Autodesk Inventor part; units mm, degrees
ref_plane "YZ Plane" through (0, 0, 0) normal (1, 0, 0) x (0, 1, 0)
ref_plane "XZ Plane" through (0, 0, 0) normal (0, 1, 0) x (-1, 0, 0)
ref_plane "XY Plane" through (0, 0, 0) normal (0, 0, 1) x (1, 0, 0)
sketch "Sketch1" plane through (0, 0, 0) normal (0, 1, 0) x (-1, 0, 0)
  circle A0 centre (0, 0) radius 14
  dimension "d0" = 28
extrude "Extrusion1" add sketch "Sketch1" along normal blind 50
sketch "Sketch2" plane through (0, 50, 0) normal (0, 1, 0) x (1, 0, 0)
  circle A0 centre (0, 0) radius 2.5
  dimension "d3" = 5
hole "Hole1" at (0, 50, 0) direction (0, -1, 0) diameter 10.106 depth 50 tip angle 118
sketch "Sketch3" plane through (0, 0, 0) normal (1, 0, 0) x (0, 1, 0)
  line L0 (50, -14) -> (50, 14)
  line L1 (50, 14.1595) -> (0, -14)
  line L2 (0, 14) -> (0, -14)
  line L3 (50, 14.1595) -> (50, -14)
  line L4 (0, 14.1595) -> (15, 14.1595)
  line L5 (15, 14.1595) -> (15, 0.0798)
  circle A0 centre (15, 0.0798) radius 2
  point P0 (0, 0)
  dimension "d11" = 15
  dimension "d12" = 4
hole "Hole2" at (0, 15, 0.0798) direction (-1, 0, 0) diameter 6.647 depth 22.2 tip angle 118
fillet "Fillet1" radius 5 1 edges at (14, 0, 0)
properties part number "FIXADOR_APOIO_ROLAMENTO"
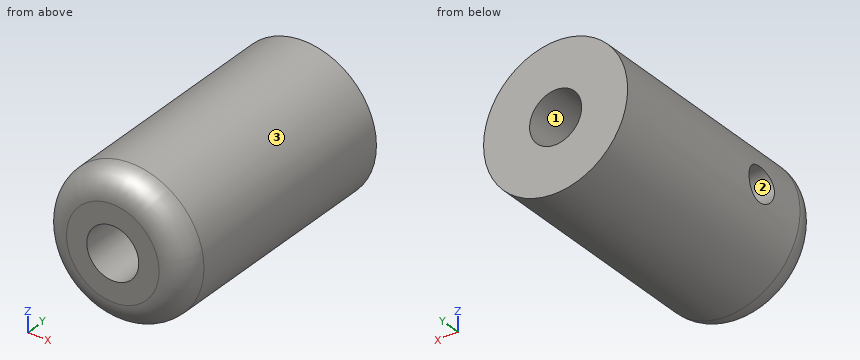
The listing builds one solid part. Answer for the finished solid, in the listing's coordinates (mm). Face numbers are marked on the shaded views. Round coordinates to 2 decimals unless told otherwise and drop trailing zeros. Order: outer loops, then holes, each group sorted by start corner. A loop starts at its lowest first (then second) coordinate and runs counter-clockwise, first axis right, second up. Notation, with made-up numbers: (31, 39.25) - (87, 39.25) arc R18 cw to (87, 56.25) - close; hole circle Ø10 at (23.25, 43). An arc over 180 degrees is marked (long way). Write item = value, one per line. Start each with the question number.
1) Straight lines are drawn through the part: L1, parallel to Z at x = 0, y = 18.5; L2, parallel to X at y = 3.5, z = -1.5; L3, parallel to Z at x = -7.5, y = 15. For each, find the intervals that lie inside material, in ascending order.
2) For a pull along X with two mould halves and no side action, classify the marked faces 1, 2 and 3 as released by +X, released by -X, zero draft, split by the parting line, or undercut.
3) Section C-C, the plane y = 24 is taken. Write down the section's boundary in (x, z).
4) Section B-B, the plane z = 0 is taken. Write down the section's boundary in (x, y).
5) Given pin 1 (6 mm diameter, centred on y = 30, z = -2.5, fed in from -X); pin 2 (4 mm diameter, centred on x = 9.5, z = 6.5, fed in from -Y); pin 3 (1 mm diameter, centred on x = -10, z = -6, fed in from -Y); pin 4 (5 mm diameter, centred on x = -3, y = 35.5, fed in from -Z), each flat-ended and moving along its own axis, determine where each tip first touches the part or whether it passes through.
6) Section D-D, the plane y = 15 is taken. Write down the section's boundary in (x, z).
7) Section A-A, the plane x = 0 is taken. Write down the section's boundary in (y, z), plus the area to 3 significant figures.
Results list:
q1.L1 = -14 to -5.05, 5.05 to 14
q1.L2 = -13.69 to -4.83, 4.83 to 13.69
q1.L3 = -11.82 to -3.24, 3.4 to 11.82
q2.face_1 = undercut
q2.face_2 = zero draft
q2.face_3 = split by the parting line
q3.outline = circle Ø28 at (0, 0); hole circle Ø10.11 at (0, 0)
q4.outline = (-14, 5) arc R5 ccw to (-9, 0) - (-5.05, 0) - (-5.05, 11.68) - (-14, 11.68) - close; (-14, 18.32) - (-5.05, 18.32) - (-5.05, 50) - (-14, 50) - close; (5.05, 0) - (9, 0) arc R5 ccw to (14, 5) - (14, 50) - (5.05, 50) - close
q5.pin_1 = -14
q5.pin_2 = 0.03
q5.pin_3 = 0.49
q5.pin_4 = -13.99
q6.outline = (-13.62, -3.24) arc R14 ccw (long way) to (-13.58, 3.4) - (-3.74, 3.4) arc R5.05 cw (long way) to (-3.87, -3.24) - close
q7.outline = (0, -9) arc R5 ccw to (5, -14) - (50, -14) - (50, -5.05) - (0, -5.05) - close; (0, 5.05) - (50, 5.05) - (50, 14) - (5, 14) arc R5 ccw to (0, 9) - close
q7.area = 884 mm^2
